Here's how the part is built. I have some questions about the finished solid (model axes, mm). A direction names the side the tool comes from. Give positions to 0.01 mm unless a question says otherwise; leave off trailing zeros. Loops run counter-clockwise (first coordinate to the right, second up) from the corner with the lowest first, then second, coordinate; pieces in that order, holes last.
Q1. If we section it at D-D (x = -50): Please give me the cut outline in (y, z).
Q2. If we section it at B-B (x = 23): Please give me the cut outline in (y, z).
Q3. Will these pins go through, and if not, where does the flat tip stop? P1, Ø10, axis at x = 18, y = 10, coming from the -Z side; P2, Ø5, axis at y = 3, z = 15.5, coming from the -X side; P3, Ø1, axis at x = 11.5, y = 9.5, coming from the +Z side; P4, Ø1.5, axis at x = 34.5, z = -34.5, coming from the -Y side.
Q4. If we section it at C-C (z = -57.5): Please give me the cut outline in (x, y), plus the area to 3 significant figures.
Q5. For faces 1 (the face through (-46.578, 4.93, -16.598)), 2 (the face through (1.448, 9.86, 54.985)), which set-ups out of +Z, -Z, +X, -X, +Y, -Y let a thin tool reach every point of the face, with its end or its side?
Q6. I need wall thicknesses on line 1 (X direction, y = 2.25, z = -15.5); line 2 (Z direction, x = 17, y = 2.25); line 3 (X direction, y = 4.5, z = 20.5). Which ranges of each line are inside material? Lowest first, please.
Q7. We'd pull the mould along X, two halves only. Please class faces 3 (the face through (-71.26, 9.86, -20.57)), 4 (the face through (-1, 20, -11)), 5 (the face through (-1.08, 4.93, -69.99)): +X half, -X half, draft (parallel to the pull), parting line (faces both ways), or undercut.
Q8. If we section it at A-A (y = 1.75): Please give me the cut outline in (x, z), plus the area to 3 significant figures.
from build123d import *

# Parameters (mm, degrees)
EXTRUDE_3_DEPTH     = 20
CUT_EXTRUDE_2_DEPTH = 10


with BuildPart() as part:
    # Sketch 1 → Extrude 3 (new body)
    # profile 1 of 6: a face of its own
    with BuildSketch(Plane(origin=(0, 0, 0), x_dir=(1, 0, 0), z_dir=(0, 1, 0))):
        with BuildLine():
            ThreePointArc((67.082039325, 33.541019662), (71.229458894, 20.760662474), (71.418701356, 7.325529194))
            ThreePointArc((71.418701356, 7.325529194), (0, -55), (-71.418701356, 7.325529194))
            ThreePointArc((-71.418701356, 7.325529194), (-71.229458894, 20.760662474), (-67.082039325, 33.541019662))
            ThreePointArc((-67.082039325, 33.541019662), (0, 75), (67.082039325, 33.541019662))
        make_face()
        with BuildLine():
            ThreePointArc((62.60990337, 31.304951685), (0, 70), (-62.60990337, 31.304951685))
            ThreePointArc((-62.60990337, 31.304951685), (-66.296498543, 19.944634184), (-66.464714064, 8.002293491))
            ThreePointArc((-66.464714064, 8.002293491), (0, -50), (66.464714064, 8.002293491))
            ThreePointArc((66.464714064, 8.002293491), (66.296498543, 19.944634184), (62.60990337, 31.304951685))
        make_face(mode=Mode.SUBTRACT)
    # profile 2 of 6: a face of its own
    with BuildSketch(Plane(origin=(0, 0, 0), x_dir=(1, 0, 0), z_dir=(0, 1, 0))):
        with BuildLine():
            ThreePointArc((62.60990337, 31.304951685), (66.296498543, 19.944634184), (66.464714064, 8.002293491))
            ThreePointArc((66.464714064, 8.002293491), (0, -50), (-66.464714064, 8.002293491))
            ThreePointArc((-66.464714064, 8.002293491), (-66.296498543, 19.944634184), (-62.60990337, 31.304951685))
            ThreePointArc((-62.60990337, 31.304951685), (0, 70), (62.60990337, 31.304951685))
        make_face()
        with BuildLine():
            ThreePointArc((53.66563146, 26.83281573), (0, 60), (-53.66563146, 26.83281573))
            ThreePointArc((-53.66563146, 26.83281573), (-56.430577839, 18.312577604), (-56.55673948, 9.355822084))
            ThreePointArc((-56.55673948, 9.355822084), (0, -40), (56.55673948, 9.355822084))
            ThreePointArc((56.55673948, 9.355822084), (56.430577839, 18.312577604), (53.66563146, 26.83281573))
        make_face(mode=Mode.SUBTRACT)
    # profile 3 of 6: a face of its own
    with BuildSketch(Plane(origin=(0, 0, 0), x_dir=(1, 0, 0), z_dir=(0, 1, 0))):
        with BuildLine():
            Line((0, 5), (0, 50))
            ThreePointArc((0, 50), (-26.286555606, 42.532540418), (-44.72135955, 22.360679775))
            ThreePointArc((-44.72135955, 22.360679775), (-46.564657136, 16.680521024), (-46.648764897, 10.709350678))
            ThreePointArc((-46.648764897, 10.709350678), (-30.957060984, -18.391595987), (0, -30))
            Line((0, -30), (0, -5))
            ThreePointArc((0, -5), (-5, 0), (0, 5))
        make_face()
    # profile 4 of 6: a face of its own
    with BuildSketch(Plane(origin=(0, 0, 0), x_dir=(1, 0, 0), z_dir=(0, 1, 0))):
        with BuildLine():
            ThreePointArc((44.72135955, 22.360679775), (26.286555606, 42.532540418), (0, 50))
            Line((0, 50), (0, 5))
            ThreePointArc((0, 5), (3.535533906, 3.535533906), (5, 0))
            ThreePointArc((5, 0), (3.535533906, -3.535533906), (0, -5))
            Line((0, -5), (0, -30))
            ThreePointArc((0, -30), (30.957060984, -18.391595987), (46.648764897, 10.709350678))
            ThreePointArc((46.648764897, 10.709350678), (46.564657136, 16.680521024), (44.72135955, 22.360679775))
        make_face()
    # profile 5 of 6: a face of its own
    with BuildSketch(Plane(origin=(0, 0, 0), x_dir=(1, 0, 0), z_dir=(0, 1, 0))):
        with BuildLine():
            ThreePointArc((53.66563146, 26.83281573), (31.543866727, 51.039048501), (0, 60))
            Line((0, 60), (0, 50))
            ThreePointArc((0, 50), (26.286555606, 42.532540418), (44.72135955, 22.360679775))
            ThreePointArc((44.72135955, 22.360679775), (46.564657136, 16.680521024), (46.648764897, 10.709350678))
            ThreePointArc((46.648764897, 10.709350678), (30.957060984, -18.391595987), (0, -30))
            Line((0, -30), (0, -40))
            ThreePointArc((0, -40), (37.532192696, -25.926026488), (56.55673948, 9.355822084))
            ThreePointArc((56.55673948, 9.355822084), (56.430577839, 18.312577604), (53.66563146, 26.83281573))
        make_face()
    # profile 6 of 6: a face of its own
    with BuildSketch(Plane(origin=(0, 0, 0), x_dir=(1, 0, 0), z_dir=(0, 1, 0))):
        with BuildLine():
            Line((0, 50), (0, 60))
            ThreePointArc((0, 60), (-31.543866727, 51.039048501), (-53.66563146, 26.83281573))
            ThreePointArc((-53.66563146, 26.83281573), (-56.430577839, 18.312577604), (-56.55673948, 9.355822084))
            ThreePointArc((-56.55673948, 9.355822084), (-37.532192696, -25.926026488), (0, -40))
            Line((0, -40), (0, -30))
            ThreePointArc((0, -30), (-30.957060984, -18.391595987), (-46.648764897, 10.709350678))
            ThreePointArc((-46.648764897, 10.709350678), (-46.564657136, 16.680521024), (-44.72135955, 22.360679775))
            ThreePointArc((-44.72135955, 22.360679775), (-26.286555606, 42.532540418), (0, 50))
        make_face()
    extrude(amount=EXTRUDE_3_DEPTH)

    # Sketch 1_4 → Cut-Extrude 2 (cut)
    # profile 1 of 3: a face of its own
    with BuildSketch(Plane(origin=(0, 0, 0), x_dir=(1, 0, 0), z_dir=(0, 1, 0))):
        with BuildLine():
            ThreePointArc((62.60990337, 31.304951685), (66.296498543, 19.944634184), (66.464714064, 8.002293491))
            ThreePointArc((66.464714064, 8.002293491), (0, -50), (-66.464714064, 8.002293491))
            ThreePointArc((-66.464714064, 8.002293491), (-66.296498543, 19.944634184), (-62.60990337, 31.304951685))
            ThreePointArc((-62.60990337, 31.304951685), (0, 70), (62.60990337, 31.304951685))
        make_face()
        with BuildLine():
            ThreePointArc((53.66563146, 26.83281573), (0, 60), (-53.66563146, 26.83281573))
            ThreePointArc((-53.66563146, 26.83281573), (-56.430577839, 18.312577604), (-56.55673948, 9.355822084))
            ThreePointArc((-56.55673948, 9.355822084), (0, -40), (56.55673948, 9.355822084))
            ThreePointArc((56.55673948, 9.355822084), (56.430577839, 18.312577604), (53.66563146, 26.83281573))
        make_face(mode=Mode.SUBTRACT)
    # profile 2 of 3: a face of its own
    with BuildSketch(Plane(origin=(0, 0, 0), x_dir=(1, 0, 0), z_dir=(0, 1, 0))):
        with BuildLine():
            Line((0, 50), (0, 60))
            ThreePointArc((0, 60), (-31.543866727, 51.039048501), (-53.66563146, 26.83281573))
            ThreePointArc((-53.66563146, 26.83281573), (-56.430577839, 18.312577604), (-56.55673948, 9.355822084))
            ThreePointArc((-56.55673948, 9.355822084), (-37.532192696, -25.926026488), (0, -40))
            Line((0, -40), (0, -30))
            ThreePointArc((0, -30), (-30.957060984, -18.391595987), (-46.648764897, 10.709350678))
            ThreePointArc((-46.648764897, 10.709350678), (-46.564657136, 16.680521024), (-44.72135955, 22.360679775))
            ThreePointArc((-44.72135955, 22.360679775), (-26.286555606, 42.532540418), (0, 50))
        make_face()
    # profile 3 of 3: a face of its own
    with BuildSketch(Plane(origin=(0, 0, 0), x_dir=(1, 0, 0), z_dir=(0, 1, 0))):
        with BuildLine():
            ThreePointArc((53.66563146, 26.83281573), (31.543866727, 51.039048501), (0, 60))
            Line((0, 60), (0, 50))
            ThreePointArc((0, 50), (26.286555606, 42.532540418), (44.72135955, 22.360679775))
            ThreePointArc((44.72135955, 22.360679775), (46.564657136, 16.680521024), (46.648764897, 10.709350678))
            ThreePointArc((46.648764897, 10.709350678), (30.957060984, -18.391595987), (0, -30))
            Line((0, -30), (0, -40))
            ThreePointArc((0, -40), (37.532192696, -25.926026488), (56.55673948, 9.355822084))
            ThreePointArc((56.55673948, 9.355822084), (56.430577839, 18.312577604), (53.66563146, 26.83281573))
        make_face()
    extrude(amount=CUT_EXTRUDE_2_DEPTH, mode=Mode.SUBTRACT)


solid = part.part
Check sheet entries:
1. outline: (0, -55.9) - (20, -55.9) - (20, 34.84) - (0, 34.84) - (0, 27.64) - (10, 27.64) - (10, -48.99) - (0, -48.99) - close
2. outline: (0, -71.39) - (20, -71.39) - (20, 51.23) - (0, 51.23) - (0, 45.93) - (10, 45.93) - (10, 24) - (0, 24) - (0, -44.4) - (10, -44.4) - (10, -66.11) - (0, -66.11) - close
3. P1: stops at z = -73.86
3. P2: stops at x = -65.5
3. P3: stops at z = 54.16
3. P4: stops at y = 0
4. outline: (-48.15, 0) - (-39.92, 0) - (-39.92, 10) - (39.92, 10) - (39.92, 0) - (48.15, 0) - (48.15, 20) - (-48.15, 20) - close
4. area: 1,130 mm2
5. face 1: -Y
5. face 2: +Z, +Y, -Y
6. line 1: x = -71.78 to -66.78, -46.72 to 46.72, 66.78 to 71.78
6. line 2: z = -73.05 to -67.9, -47.02 to 26.82, 47.81 to 52.97
6. line 3: x = -61.51 to -55.57, -28.36 to 28.36, 55.57 to 61.51
7. face 3: -X half
7. face 4: draft
7. face 5: undercut
8. outline: (-71.42, -7.33) arc R45 ccw to (-67.08, -33.54) arc R75 ccw to (67.08, -33.54) arc R45 ccw to (71.42, -7.33) arc R72.08 ccw to start; (-46.65, -10.71) arc R20 ccw to (-44.72, -22.36) arc R50 ccw to (44.72, -22.36) arc R20 ccw to (46.65, -10.71) arc R47.08 ccw to start; hole (-66.46, -8) arc R40 ccw to (-62.61, -31.3) arc R70 ccw to (62.61, -31.3) arc R40 ccw to (66.46, -8) arc R67.08 ccw to start; hole circle Ø10 at (0, 0)
8. area: 7,710 mm2
